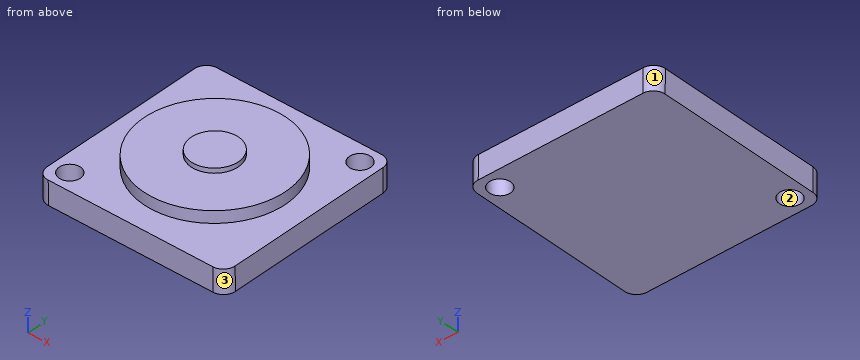
from build123d import *

# Parameters (mm, degrees)
BOSS_EXTRUDE2_DEPTH      = 4.999462447
BOSS_EXTRUDE2_DEPTH_BACK = 0.0001
SKETCH4_W                = 40
SKETCH4_H                = 40
SKETCH6_R                = 15
BOSS_EXTRUDE3_DEPTH      = 2.5
SKETCH7_R                = 5
BOSS_EXTRUDE4_DEPTH      = 1
SKETCH9_R                = 2.25
CUT_EXTRUDE1_DEPTH       = 5
SKETCH10_R               = 2.25
CUT_EXTRUDE2_DEPTH       = 5
FILLET2_R                = 2.5
BODY_MOVE_COPY2_ANGLE    = 90.001090824


with BuildPart() as part:
    # Sketch4 → Boss-Extrude2 (new, two sides: drawn at the far end of the back side and taken through both)
    with BuildSketch(Plane.XY.offset(-BOSS_EXTRUDE2_DEPTH_BACK)):
        Rectangle(SKETCH4_W, SKETCH4_H)
    extrude(amount=BOSS_EXTRUDE2_DEPTH + BOSS_EXTRUDE2_DEPTH_BACK)

    # Sketch6 → Boss-Extrude3 (add)
    with BuildSketch(Plane.XY.offset(4.999462447)):
        Circle(SKETCH6_R)
    extrude(amount=BOSS_EXTRUDE3_DEPTH)

    # Sketch7 → Boss-Extrude4 (add)
    with BuildSketch(Plane.XY.offset(7.499462447)):
        Circle(SKETCH7_R)
    extrude(amount=BOSS_EXTRUDE4_DEPTH)

    # Sketch9 → Cut-Extrude1 (cut)
    with BuildSketch(Plane.XY.offset(4.999462447)):
        with Locations((-16.263, 16.263)):
            Circle(SKETCH9_R)
    extrude(amount=-CUT_EXTRUDE1_DEPTH, mode=Mode.SUBTRACT)

    # Sketch10 → Cut-Extrude2 (cut)
    with BuildSketch(Plane.XY.offset(4.999462447)):
        with Locations((16.263, -16.263)):
            Circle(SKETCH10_R)
    extrude(amount=-CUT_EXTRUDE2_DEPTH, mode=Mode.SUBTRACT)

    # Fillet2
    fillet2_edges = [part.edges().sort_by_distance(p)[0] for p in [
        (20, -20, 2.499681224),
        (-20, -20, 2.499681224),
        (-20, 20, 2.499681224),
        (20, 20, 2.499681224),
    ]]
    fillet(fillet2_edges, radius=FILLET2_R)


with BuildPart() as part_1:
    # Body-Move/Copy2: moved
    add(part.part.moved(Location((0, 0, 0))).rotate(Axis((0.018337793, 0.018337793, 0.000160028), (0.004363267749989983, 0.004363267749984885, -0.9999809617133137)), BODY_MOVE_COPY2_ANGLE))


solid = part_1.part
Here's how the part is built. I have some questions about the finished solid (model axes, mm). Face numbers are marked on the shaded views. Round coordinates to 2 decimals unless told otherwise and drop trailing zeros. Loops run counter-clockwise (first coordinate to the right, second up) from the corner with the lowest first, then second, coordinate; pieces in that order, holes last. Notation, with made-up numbers: (58, 52.5) -> (82, 52.5) arc R32 cw to (82, 85.5) -> close; hole circle Ø7 at (33, -29.5). An arc over 180 degrees is marked (long way). Write each question's results on one line, items separated by ' | '.
(1) If we section it at A-A, the plane x = 12: List the corners of the cut face in (y, z) for me, then the cut area to 3 significant figures.
Worked answers:
outline: (-20.01, 4.82) -> (-19.96, -0.17) -> (20.04, 0.17) -> (19.99, 5.17) -> (8.99, 5.08) -> (8.97, 7.58) -> (-9.03, 7.42) -> (-9.01, 4.92) -> close | area: 245 mm2
(2) If we section it at C-C, the plane x = 3: List the corners of the cut face in (y, z) for me, then the cut area to 3 significant figures.
Worked answers:
outline: (-20.01, 4.82) -> (-19.96, -0.17) -> (20.04, 0.17) -> (19.99, 5.17) -> (14.69, 5.13) -> (14.67, 7.63) -> (3.97, 7.53) -> (3.96, 8.53) -> (-4.04, 8.46) -> (-4.03, 7.46) -> (-14.73, 7.37) -> (-14.7, 4.87) -> close | area: 281 mm2
(3) If we section it at B-B, the plane z = 1.5: Give the number of separate pieces and of enclosed holes in the cut face, then the cut area to 3 significant figures.
Worked answers:
separate pieces: 1 | enclosed holes: 2 | area: 1,560 mm2
(4) For P1, Ø6, axis at x = 9, y = -2, coming from the +Z side; P2, Ø1.5, axis at x = 8, y = -14.5, coming from the +Z side; P3, Ø4, axis at x = 10, y = -1, coming from the -Z side, each with a flat end and sliding along its axis, tell me the tip position at first contact or that it passes through.
Worked answers:
P1: z = 7.51 | P2: z = 4.88 | P3: z = -0.03
(5) If we section it at D-D, the plane x = -11: List the corners of the cut face in (y, z) for me.
Worked answers:
outline: (-20.01, 4.82) -> (-19.96, -0.17) -> (20.04, 0.17) -> (19.99, 5.17) -> (10.19, 5.09) -> (10.17, 7.59) -> (-10.23, 7.41) -> (-10.2, 4.91) -> close
(6) We'd pull the mould along X, two halves only. Please class the marked faces 1, 2 and 3: released by +X, released by -X, zero draft, split by the parting line, or undercut.
Worked answers:
face 1: released by -X | face 2: undercut | face 3: released by +X
(7) If I drill on L1, parallel to Z at x = 3, y = -16.5; L2, parallel to Y at x = 9.5, z = 4; L3, parallel to Z at x = 2, y = -17.5, over which ranges is the centre line in solid material (lowest first)?
Worked answers:
L1: -0.14 to 4.86 | L2: -20 to 20 | L3: -0.15 to 4.85
